Solid Edge part; units mm, degrees
sketch "Sketch1" plane through (0, 0, 0) normal (0, -1, 0) x (1, 0, 0)
  circle A0 centre (0, 0) radius 6.5
extrude "Protrusion1" add sketch "Sketch1" against normal blind 15
sketch "Sketch2" plane through (0, 0, 0) normal (0, -1, 0) x (1, 0, 0)
  circle A0 centre (0, 0) radius 6.5
extrude "holder" add sketch "Sketch2" along normal blind 2
sketch "Sketch3" plane through (0, -2, 0) normal (0, -1, 0) x (1, 0, 0)
  circle A0 centre (0, 0) radius 4
extrude "Cutout1" cut sketch "Sketch3" against normal through all
sketch "Sketch4" plane through (0, -2, 0) normal (0, -1, 0) x (1, 0, 0)
  circle A0 centre (0, 0) radius 5.5
extrude "Cutout2" cut sketch "Sketch4" against normal blind 15.5
Verification items for the finished model (mm, model axes). A direction names the side the tool comes from. Coordinates: 2 decimals unless noted, no trailing zeros. Order: outer loops, then holes, each group sorted by start corner. A loop starts at its lowest first (then second) coordinate and runs counter-clockwise, first axis right, second up. Notation, with made-up numbers: M 45,31.5 L 69,31.5 A17 ccw 69,56.5 Z; hole C 87.25,-2 d1. An arc over 180 degrees is marked long. Return JSON: item names as keys, results as strings.
1) Access from +Z, -Z, +X, -X, +Y, -Y to the whole of each face (thin tool, end or side, straight path). Record for faces 5 (the flat face through (3, -2, 5)), 6 (the cylindrical face through (-1.19, 5.64, -5.37)).
Answer list:
{"face 5": "+Z, -Z, +X, -X, -Y", "face 6": "-Y"}
2) Gauge pin test, flat ends, axial feed: pin 1 (1.5 mm diameter, centred on x = -4, z = -1, fed in from -Y); pin 2 (1 mm diameter, centred on y = 12.5, z = -4, fed in from -X); pin 3 (1 mm diameter, centred on y = 12.5, z = -5, fed in from +X); pin 4 (5.5 mm diameter, centred on x = -2, z = -2.5, fed in from -Y). Record the tip position at first contact, or that the pin passes through.
Answer list:
{"pin 1": "y = 13.5", "pin 2": "x = -5.48", "pin 3": "x = 4.69", "pin 4": "y = -2"}
3) Thickness scan on L1, parallel to Z at x = 0, y = 14.2; L2, parallel to Z at x = 0, y = 4.75; L3, parallel to X at y = 7.5, z = -1.5. Record the ranges inside material, lowest first. Write a range as [from, to].
Answer list:
{"L1": "[-6.5, -4], [4, 6.5]", "L2": "[-6.5, -5.5], [5.5, 6.5]", "L3": "[-6.32, -5.29], [5.29, 6.32]"}
4) Cross-section at A-A, the plane z = 0. Record the boundary of the cut face in (x, y), and give its area (3 significant figures).
Answer list:
{"outline": "M -6.5,-2 L -5.5,-2 L -5.5,13.5 L -4,13.5 L -4,15 L -6.5,15 Z; M 4,13.5 L 5.5,13.5 L 5.5,-2 L 6.5,-2 L 6.5,15 L 4,15 Z", "area": "38.5 mm2"}
5) Release check for a two-part mould opening along Z. For faces 1 (the flat face through (3, 15, -3)), 2 (the cylindrical face through (-0.867, 14.24, -3.905)), 3 (the flat face through (-2, 13.5, 4)), 4 (the cylindrical face through (-5.158, 6.381, -3.955)) record: +Z half, -Z half, draft (parallel to the pull), parting line (faces both ways), or undercut.
Answer list:
{"face 1": "draft", "face 2": "undercut", "face 3": "undercut", "face 4": "parting line"}
6) Cross-section at D-D, the plane x = -4.25. Record the boundary of the cut face in (y, z).
Answer list:
{"outline": "M -2,-4.92 L 15,-4.92 L 15,4.92 L -2,4.92 L -2,3.49 L 13.5,3.49 L 13.5,-3.49 L -2,-3.49 Z"}
7) Cross-section at C-C, the plane y = 8. Record the boundary of the cut face in (x, z), and give its area (3 significant figures).
Answer list:
{"outline": "C 0,0 d13; hole C 0,0 d11", "area": "37.7 mm2"}
8) Cross-section at B-B, the plane x = 0. Record the boundary of the cut face in (y, z), and give its area (3 significant figures).
Answer list:
{"outline": "M -2,-6.5 L 15,-6.5 L 15,-4 L 13.5,-4 L 13.5,-5.5 L -2,-5.5 Z; M -2,5.5 L 13.5,5.5 L 13.5,4 L 15,4 L 15,6.5 L -2,6.5 Z", "area": "38.5 mm2"}
